CAD build for the part. Positions are in the model's coordinates, mm. A direction names the side the tool comes from. Round coordinates to 2 decimals unless told otherwise and drop trailing zeros. Order: outer loops, then holes, each group sorted by start corner. A loop starts at its lowest first (then second) coordinate and runs counter-clockwise, first axis right, second up. Notation, with made-up numbers: (34, -25.75) -> (49, -25.75) arc R21 ccw to (49, -10.75) -> close; hole circle Ø4 at (12.5, 17.5). An arc over 180 degrees is marked (long way). Return JSON: item names as keys, results as strings. Group by question number.
Q1. Cut at A-A (x = 10). Write the cut outline in (y, z), then the cut area to 3 significant figures.
Q2. Which spindle directions (+Z, -Z, +X, -X, +Y, -Y) get a long thin tool onto all of the face, cutting with end or side? Do faces 1 (the flat face through (16, 11, 2)), 2 (the flat face through (4, 10, 2)), 3 (the flat face through (4, -2, 2)), 4 (the flat face through (18, 0, 2)). Say none if no direction does.
Q3. Probe line 1 along Y through (x, z) = (10, 2.9); line 2 along X through (y, z) = (16, 1.15); line 3 along X through (y, z) = (-0.5, 3.4). List the from-to ranges inside material, lowest first.
Q4. Cut at D-D (x = 16.75). Write the cut outline in (y, z).
Q5. Flat gauge pins, fed straight in: pin 1 (1.2 mm diameter, centred on y = -2, z = 3, fed in from +X); pin 2 (2 mm diameter, centred on x = 2.5, z = 2, fed in from -Y); pin 3 (1 mm diameter, centred on y = 5.5, z = 2.5, fed in from -X). Where does each tip first touch, or does it go through?
Q6. Cut at C-C (z = 1). Write the cut outline in (x, y).
Q7. Mould opens along Y. For faces 5 (the cylindrical face through (12.71, 18.26, 1.97)), 6 (the flat face through (2, 0, 2)), 7 (the flat face through (16, -2, 2)) say: +Y half, -Y half, draft (parallel to the pull), parting line (faces both ways), or undercut.
Q8. Cut at B-B (y = 14). Write the cut outline in (x, z), then the cut area to 3 significant figures.
from build123d import *

# Parameters (mm, degrees)
SKETCH_1_R      = 5.05
EXTRUDE_1_DEPTH = 4


with BuildPart() as part:
    # Эскиз1 → Бобышка-Вытянуть1 (new body)
    with BuildSketch(Plane.XY):
        with BuildLine():
            Line((0, 0), (0, 4))
            Line((0, 4), (4, 4))
            Line((4, 4), (4, 8))
            Line((4, 8), (4, 17))
            ThreePointArc((4, 17), (4.878679656, 19.121320344), (7, 20))
            Line((7, 20), (13, 20))
            ThreePointArc((13, 20), (15.121320344, 19.121320344), (16, 17))
            Line((16, 17), (16, 8))
            Line((16, 8), (16, 4))
            Line((16, 4), (20, 4))
            Line((20, 4), (20, 0))
            Line((20, 0), (16, 0))
            Line((16, 0), (16, -4))
            Line((16, -4), (4, -4))
            Line((4, -4), (4, 0))
            Line((4, 0), (0, 0))
        make_face()
        with Locations((10, 14)):
            Circle(SKETCH_1_R, mode=Mode.SUBTRACT)
    extrude(amount=EXTRUDE_1_DEPTH)


solid = part.part
Solution:
{
 "1": {"outline": "(-4, 0) -> (8.95, 0) -> (8.95, 4) -> (-4, 4) -> close; (19.05, 0) -> (20, 0) -> (20, 4) -> (19.05, 4) -> close", "area": "55.6 mm²"},
 "2": {"face 1": "+Z, -Z, +X, +Y", "face 2": "+Z, -Z, -X, +Y", "face 3": "+Z, -Z, -X, -Y", "face 4": "+Z, -Z, +X, -Y"},
 "3": {"line 1": "y = -4 to 8.95, 19.05 to 20", "line 2": "x = 4 to 5.36, 14.64 to 16", "line 3": "x = 4 to 16"},
 "4": {"outline": "(0, 0) -> (4, 0) -> (4, 4) -> (0, 4) -> close"},
 "5": {"pin 1": "stops at x = 16", "pin 2": "stops at y = 0", "pin 3": "stops at x = 4"},
 "6": {"outline": "(0, 0) -> (4, 0) -> (4, -4) -> (16, -4) -> (16, 0) -> (20, 0) -> (20, 4) -> (16, 4) -> (16, 17) arc R3 ccw to (13, 20) -> (7, 20) arc R3 ccw to (4, 17) -> (4, 4) -> (0, 4) -> close; hole circle Ø10.1 at (10, 14)"},
 "7": {"face 5": "undercut", "face 6": "-Y half", "face 7": "draft"},
 "8": {"outline": "(4, 0) -> (4.95, 0) -> (4.95, 4) -> (4, 4) -> close; (15.05, 0) -> (16, 0) -> (16, 4) -> (15.05, 4) -> close", "area": "7.60 mm²"}
}
